Read the model definition and answer for the solid it produces. Units are mm, in the model's axes. A direction names the side the tool comes from. Coordinates: 2 decimals unless noted, no trailing zeros. Loops run counter-clockwise (first coordinate to the right, second up) from the corner with the lowest first, then second, coordinate; pieces in that order, holes last. Notation, with made-up numbers: M 49.5,-20 L 86.5,-20 A20 ccw 86.5,8 Z; hole C 56.25,-15 d10. An arc over 180 degrees is marked long. One line per item, written item: value. Start each with the question number.
1. The part is cut by section A-A (z = 137.5). Write down the section's boundary in (x, y), then the cut area to 4 significant figures.
2. The part is cut by section C-C (y = 74.5). Write down the section's boundary in (x, z).
3. The part is cut by section D-D (x = -75.5). Write down the section's boundary in (y, z), then the cut area to 3 significant figures.
4. Consider probe 1 along X at (y, z) = (38.5, 208); probe 2 along X at (y, z) = (102.5, 224); probe 3 along Z at (x, y) = (-12.5, 41). Determine where each line is inside the solid, lowest interval first.
5. For faces 1 (the face through (104.717, 41, 173)), 2 (the face through (29, 64.084, 330)), 3 (the face through (-45.283, 42, 173)), 4 (the face through (31, 109.084, 129)), determine the directions among +Z, -Z, +X, -X, +Y, -Y from which every point of the face is accessible in a straight line to the end or side of a thin tool.
6. The part is cut by section B-B (x = -10). Write down the section's boundary in (y, z), then the cut area to 3 significant figures.
7. Flat-ended cylindrical pins translate along their axes: pin 1 (1 mm diameter, centred on x = 87.5, y = 99, fed in from +Z); pin 2 (4 mm diameter, centred on y = 49.5, z = 45, fed in from +X); pin 3 (13.5 mm diameter, centred on y = 40, z = 116.5, fed in from -X). Find the tip coordinate at first contact, or state that the pin passes through.
Autodesk Inventor part; units mm, degrees
ref_plane "YZ Plane" through (0, 0, 0) normal (1, 0, 0) x (0, 1, 0)
ref_plane "XZ Plane" through (0, 0, 0) normal (0, 1, 0) x (-1, 0, 0)
ref_plane "XY Plane" through (0, 0, 0) normal (0, 0, 1) x (1, 0, 0)
sketch "Эскиз2" plane through (0, 0, 0) normal (0, 0, 1) x (1, 0, 0)
  line L0 (104.717, 109.0836) -> (-45.283, 109.0836)
  line L1 (-45.283, 109.0836) -> (-45.283, 19.0836)
  line L2 (-45.283, 19.0836) -> (104.717, 19.0836)
  line L3 (104.717, 19.0836) -> (104.717, 109.0836)
  line L4 (-95.283, 19.0836) -> (154.717, 19.0836)
  line L5 (154.717, 19.0836) -> (154.717, 109.0836)
  line L6 (154.717, 109.0836) -> (-95.283, 109.0836)
  line L7 (-95.283, 109.0836) -> (-95.283, 19.0836)
  line L8 (154.717, 19.0836) -> (104.717, 19.0836)
  line L9 (104.717, 19.0836) -> (104.717, -10.9164)
  line L10 (104.717, -10.9164) -> (154.717, -10.9164)
  line L11 (154.717, -10.9164) -> (154.717, 19.0836)
  line L12 (-45.283, 19.0836) -> (-95.283, 19.0836)
  line L13 (-95.283, 19.0836) -> (-95.283, -10.9164)
  line L14 (-95.283, -10.9164) -> (-45.283, -10.9164)
  line L15 (-45.283, -10.9164) -> (-45.283, 19.0836)
  line L16 (-45.283, 64.0836) -> (-95.283, 64.0836)
  line L17 (-95.283, 64.0836) -> (-45.283, 109.0836)
  line L18 (104.717, 64.0836) -> (154.717, 64.0836)
  line L19 (154.717, 64.0836) -> (104.717, 109.0836)
  point P0 (0, 0)
  dimension "d0" = 150
  dimension "d1" = 50
  dimension "d2" = 50
  dimension "d3" = 30
  dimension "d4" = 90
  dimension "d5" = 0
  dimension "d6" = 0
extrude "Выдавливание1" add sketch "Эскиз2" along normal blind 350 contours L3 L2 L1 L0 | L19 L18 L3 | L1 L16 L17
sketch "Эскиз3" plane through (-45.283, 19.0836, 0) normal (-1, 0, 0) x (0, 0, 1)
  line L0 (0, 0) -> (350, 0)
  line L1 (296.6019, 0) -> (349.571, 44.6384)
  line L2 (350, 45) -> (350, 0)
  line L3 (349.571, 44.6384) -> (350, 45)
  line L4 (350, 45) -> (308.6701, 45)
  line L5 (0, 45) -> (350, 45)
  line L6 (308.6701, 45) -> (261.5284, 90)
  line L7 (0, 90) -> (350, 90)
  line L8 (0, 45) -> (0, 90)
  line L9 (350, 0) -> (0, 0)
  line L10 (0, 0) -> (0, 90)
  line L11 (0, 90) -> (350, 90)
  line L12 (350, 90) -> (350, 0)
  point P0 (0, -19.0836)
extrude "Выдавливание2" cut sketch "Эскиз3" against normal mid plane 1000 contours L1 L3 L2 L0 | L6 L7 L12 L4
properties part number "пример корпуса 1"
Answer block:
1. outline: M -95.28,64.08 L -45.28,64.08 L -45.28,19.08 L 104.72,19.08 L 104.72,64.08 L 154.72,64.08 L 104.72,109.08 L -45.28,109.08 Z
1. area: 15,750 mm2
2. outline: M -83.71,0 L 143.14,0 L 143.14,297.76 L -83.71,297.76 Z
3. outline: M 64.08,0 L 81.89,0 L 81.89,290.02 L 64.08,308.67 Z
3. area: 5,330 mm2
4. probe 1: x = -45.28 to 104.72
4. probe 2: x = -52.6 to 112.03
4. probe 3: z = 0 to 322.61
5. face 1: +Z, -Z, +X, -Y
5. face 2: +Z, +X, -X, +Y
5. face 3: +Z, -Z, -X, -Y
5. face 4: +Z, -Z, +X, -X, +Y
6. outline: M 19.08,0 L 109.08,0 L 109.08,261.53 L 64.08,308.67 L 64.08,350 L 63.72,349.57 L 19.08,296.6 Z
6. area: 27,400 mm2
7. pin 1: stops at z = 272.62
7. pin 2: stops at x = 104.72
7. pin 3: stops at x = -45.28
